from build123d import *

# Parameters (mm, degrees)
SKETCH1_W           = 28
SKETCH1_H           = 28
BOSS_EXTRUDE1_DEPTH = 8.449682579
CUT_EXTRUDE1_DEPTH  = 41.489469442
SKETCH3_W           = 50
SKETCH3_H           = 21
CUT_EXTRUDE2_DEPTH  = 4
SKETCH11_R          = 1.45
BOSS_EXTRUDE2_DEPTH = 4
SKETCH13_R          = 2.4
CUT_EXTRUDE5_DEPTH  = 41.489469442
BOSS_EXTRUDE3_REACH = 42.489
SKETCH14_R          = 6.4
SKETCH14_R_2        = 2.4
SKETCH15_R          = 1.4
CUT_EXTRUDE6_DEPTH  = 50.476186927
SKETCH16_R          = 1.4
CUT_EXTRUDE7_DEPTH  = 50.476187084
SKETCH18_W          = 30
SKETCH18_H          = 21
CUT_EXTRUDE8_DEPTH  = 4


with BuildPart() as part:
    # Sketch1 → Boss-Extrude1 (new body)
    with BuildSketch(Plane(origin=(0, 0, 0), x_dir=(1, 0, 0), z_dir=(0, 1, 0))):
        with Locations((14, 14)):
            Rectangle(SKETCH1_W, SKETCH1_H)
    extrude(amount=BOSS_EXTRUDE1_DEPTH)

    # Sketch2 → Cut-Extrude1 (cut, through all)
    with BuildSketch(Plane.XY):
        Polygon((0, 8.449682579), (28, 6), (28, 8.449682579), align=None)
    extrude(amount=-CUT_EXTRUDE1_DEPTH, mode=Mode.SUBTRACT)

    # Sketch3 → Cut-Extrude2 (cut)
    with BuildSketch(Plane(origin=(0.733635991, 8.385497746, 0), x_dir=(0.9961946980917455, -0.08715574274765811, 0), z_dir=(0.08715574274765811, 0.9961946980917455, 0))):
        with Locations((24.263561639, 14)):
            Rectangle(SKETCH3_W, SKETCH3_H)
    extrude(amount=-CUT_EXTRUDE2_DEPTH, mode=Mode.SUBTRACT)

    # Sketch11 → Boss-Extrude2 (add)
    with BuildSketch(Plane(origin=(0.38501302, 4.400718954, 0), x_dir=(0.9961946980917457, -0.08715574274765812, 0), z_dir=(0.08715574274765812, 0.9961946980917457, 0))):
        with Locations((4.666994019, 21)):
            Circle(SKETCH11_R)
        with Locations((4.666994019, 7)):
            Circle(SKETCH11_R)
    extrude(amount=BOSS_EXTRUDE2_DEPTH)

    # Sketch13 → Cut-Extrude5 (cut, through all)
    with BuildSketch(Plane.XZ):
        Circle(SKETCH13_R)
        with Locations((28, 0)):
            Circle(SKETCH13_R)
        with Locations((28, -28)):
            Circle(SKETCH13_R)
        with Locations((0, -28)):
            Circle(SKETCH13_R)
    extrude(amount=-CUT_EXTRUDE5_DEPTH, mode=Mode.SUBTRACT)

    # Boss-Extrude3: up to this plane
    boss_extrude3_end = Plane(origin=(0, 8.449682579, -28), z_dir=(-0.08715574274765814, -0.9961946980917457, 0))
    # Sketch14 → Boss-Extrude3 (add, up to the surface)
    with BuildSketch(Plane.XZ, mode=Mode.PRIVATE) as boss_extrude3_sk1:
        Circle(SKETCH14_R)
        with Locations(Location((0, 0, 0), (0, 0, 270))):
            Circle(SKETCH14_R_2, mode=Mode.SUBTRACT)
    boss_extrude3_tool1 = split(extrude(boss_extrude3_sk1.sketch, amount=-BOSS_EXTRUDE3_REACH, mode=Mode.PRIVATE), bisect_by=boss_extrude3_end, keep=Keep.BOTH, mode=Mode.PRIVATE)
    add(boss_extrude3_tool1.solids().sort_by_distance((-6.218981, 0, 0))[0])
    # Sketch14 → Boss-Extrude3 (add, up to the surface)
    with BuildSketch(Plane.XZ, mode=Mode.PRIVATE) as boss_extrude3_sk2:
        with Locations((28, 0)):
            Circle(SKETCH14_R)
        with Locations(Location((28, 0, 0), (0, 0, 270))):
            Circle(SKETCH14_R_2, mode=Mode.SUBTRACT)
    boss_extrude3_tool2 = split(extrude(boss_extrude3_sk2.sketch, amount=-BOSS_EXTRUDE3_REACH, mode=Mode.PRIVATE), bisect_by=boss_extrude3_end, keep=Keep.BOTH, mode=Mode.PRIVATE)
    add(boss_extrude3_tool2.solids().sort_by_distance((21.781019, 0, 0))[0])
    # Sketch14 → Boss-Extrude3 (add, up to the surface)
    with BuildSketch(Plane.XZ, mode=Mode.PRIVATE) as boss_extrude3_sk3:
        with Locations((28, -28)):
            Circle(SKETCH14_R)
        with Locations(Location((28, -28, 0), (0, 0, 270))):
            Circle(SKETCH14_R_2, mode=Mode.SUBTRACT)
    boss_extrude3_tool3 = split(extrude(boss_extrude3_sk3.sketch, amount=-BOSS_EXTRUDE3_REACH, mode=Mode.PRIVATE), bisect_by=boss_extrude3_end, keep=Keep.BOTH, mode=Mode.PRIVATE)
    add(boss_extrude3_tool3.solids().sort_by_distance((21.781019, 0, -28))[0])
    # Sketch14 → Boss-Extrude3 (add, up to the surface)
    with BuildSketch(Plane.XZ, mode=Mode.PRIVATE) as boss_extrude3_sk4:
        with Locations((0, -28)):
            Circle(SKETCH14_R)
        with Locations(Location((0, -28, 0), (0, 0, 270))):
            Circle(SKETCH14_R_2, mode=Mode.SUBTRACT)
    boss_extrude3_tool4 = split(extrude(boss_extrude3_sk4.sketch, amount=-BOSS_EXTRUDE3_REACH, mode=Mode.PRIVATE), bisect_by=boss_extrude3_end, keep=Keep.BOTH, mode=Mode.PRIVATE)
    add(boss_extrude3_tool4.solids().sort_by_distance((-6.218981, 0, -28))[0])

    # Sketch15 → Cut-Extrude6 (cut, through all)
    with BuildSketch(Plane(origin=(0, 0, -28), x_dir=(-1, 0, 0), z_dir=(0, 0, -1))):
        with Locations(Location((-28, 3, 0), (0, 0, 270))):
            Circle(SKETCH15_R)
        with Locations(Location((0, 3, 0), (0, 0, 90))):
            Circle(SKETCH15_R)
    extrude(amount=CUT_EXTRUDE6_DEPTH, mode=Mode.SUBTRACT)

    # Sketch16 → Cut-Extrude7 (cut, through all)
    with BuildSketch(Plane.XY):
        with Locations(Location((0, 3, 0), (0, 0, 90))):
            Circle(SKETCH16_R)
        with Locations(Location((28, 3, 0), (0, 0, 270))):
            Circle(SKETCH16_R)
    extrude(amount=CUT_EXTRUDE7_DEPTH, mode=Mode.SUBTRACT)

    # Sketch18 → Cut-Extrude8 (cut)
    with BuildSketch(Plane(origin=(0.733635991, 8.385497746, 0), x_dir=(0.9961946980917455, -0.08715574274765811, 0), z_dir=(0.08715574274765811, 0.9961946980917455, 0))):
        with BuildLine():
            Line((4.992154967, 24.5), (-0.386483707, 24.5))
            Line((-0.386483707, 24.5), (-0.386483707, 21.6))
            add(Edge.make_bspline(
                [(-0.386483707, 21.6), (3.090616042, 21.6), (4.992154967, 24.5)],
                knots=[4.71238898, 4.71238898, 4.71238898, 5.704558256, 5.704558256, 5.704558256], degree=2, weights=[1, 0.879452955, 1]))
        make_face()
        with Locations((21.991878416, 14)):
            Rectangle(SKETCH18_W, SKETCH18_H)
        with BuildLine():
            Line((-0.386483707, 6.4), (-0.386483707, 3.5))
            Line((-0.386483707, 3.5), (4.992154967, 3.5))
            add(Edge.make_bspline(
                [(4.992154967, 3.5), (3.090616042, 6.4), (-0.386483707, 6.4)],
                knots=[0.578627051, 0.578627051, 0.578627051, 1.570796327, 1.570796327, 1.570796327], degree=2, weights=[1, 0.879452955, 1]))
        make_face()
    extrude(amount=-CUT_EXTRUDE8_DEPTH, mode=Mode.SUBTRACT)


solid = part.part
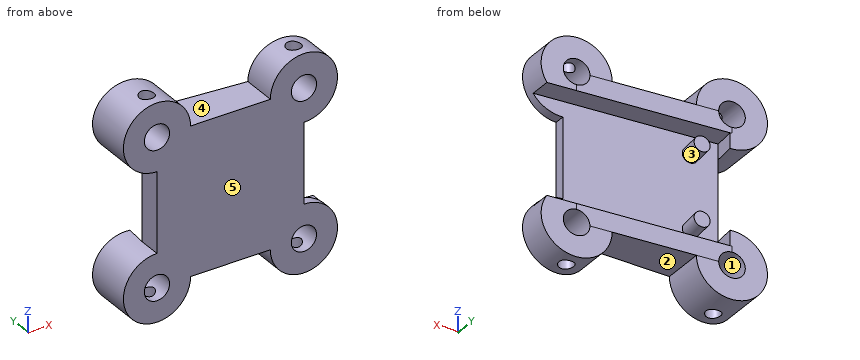
Geometry check sheet. Reference: the model listing, model coordinates, mm. Face numbers are marked on the shaded views. A direction names the side the tool comes from. Round coordinates to 2 decimals unless told otherwise and drop trailing zeros. Write each loop counter-clockwise with the first axis right and the second up, starting at its lowest first coordinate (ties: lowest second). Pieces come first, ordered by that corner, then holes. Notation, with made-up numbers: (25.25, 22) -> (45.25, 22) arc R3 cw to (45.25, 26) -> close; hole circle Ø3 at (65.25, -27.5). An arc over 180 degrees is marked (long way). One line per item, written item: value. Start each with the question number.
(1) Cross-section at C-C, the plane x = 8. Record the cut outline in (y, z).
(2) Scan lines: line 1 (Z direction, x = 28, y = 3); line 2 (X direction, y = 3, z = 3.45); line 3 (Z direction, x = 15.5, y = 6.5). Record each from-to range of solid material in increasing order. Write a range as [from, to].
(3) Go/stop test with flat-tipped pins: pin 1 Ø2 at (x, z) = (20, -29.5) entering from -Y; pin 2 Ø0.6 at (y, z) = (0.5, -16.5) entering from +X; pin 3 Ø5 at (x, z) = (3.5, -4.5) entering from +Y; pin 4 Ø3.5 at (y, z) = (1.5, -14.5) entering from -X. Record where each tip stops, or that it passes through.
(4) Access from +Z, -Z, +X, -X, +Y, -Y to the whole of each face (thin tool, end or side, straight path). Record for the marked faces 1 and 2.
(5) Cross-section at D-D, the plane x = 24. Record the cut outline in (y, z).
(6) Cross-section at B-B, the plane y = 2.5. Record the cut outline in (x, z).
(7) Cross-section at A-A, the plane z = -14. Record the cut outline in (x, y).
(8) Draft check along Y on the marked faces 3, 4 and 5. Enter one of: +Y half, -Y half, draft (parallel to the pull), parting line (faces both ways), or undercut.
Answer:
1. outline: (0, -28) -> (7.75, -28) -> (7.75, -24.5) -> (3.73, -24.5) -> (3.73, -3.5) -> (7.75, -3.5) -> (7.75, 0) -> (0, 0) -> close
2. line 1: [-25.6, -24.5], [-3.5, -2.4]
2. line 2: [-5.39, -1.4], [1.4, 5.39], [22.61, 26.6], [29.4, 33.39]
2. line 3: [-28, -24.5], [-3.5, 0]
3. pin 1: through
3. pin 2: x = 28
3. pin 3: y = 8.34
3. pin 4: x = 0
4. face 1: +Y, -Y
4. face 2: -Z, +Y, -Y
5. outline: (0, -33) -> (6.35, -33) -> (6.35, -24.5) -> (2.33, -24.5) -> (2.33, -3.5) -> (6.35, -3.5) -> (6.35, 5) -> (0, 5) -> close
6. outline: (-1.31, -34.26) -> (-1.31, -30.01) arc R2.4 cw (long way) to (1.31, -30.01) -> (1.31, -34.26) arc R6.4 ccw to (6.4, -28) -> (21.6, -28) arc R6.4 ccw to (26.69, -34.26) -> (26.69, -30.01) arc R2.4 cw (long way) to (29.31, -30.01) -> (29.31, -34.26) arc R6.4 ccw to (33.36, -24.5) -> (22.11, -24.5) -> (22.11, -3.5) -> (33.36, -3.5) arc R6.4 ccw to (29.31, 6.26) -> (29.31, 2.01) arc R2.4 cw (long way) to (26.69, 2.01) -> (26.69, 6.26) arc R6.4 ccw to (21.6, 0) -> (6.4, 0) arc R6.4 ccw to (1.31, 6.26) -> (1.31, 2.01) arc R2.4 cw (long way) to (-1.31, 2.01) -> (-1.31, 6.26) arc R6.4 ccw to (0, -6.4) -> (0, -21.6) arc R6.4 ccw to start
7. outline: (0, 0) -> (28, 0) -> (28, 1.98) -> (0, 4.43) -> close
8. face 3: undercut
8. face 4: draft
8. face 5: -Y half
